```python
from build123d import *

# Parameters (mm, degrees)
SKETCH_1_R          = 6
EXTRUDE_1_DEPTH     = 19
CUT_EXTRUDE_1_DEPTH = 82.836727696


with BuildPart() as part:
    # Эскиз1 → Бобышка-Вытянуть1 (new, symmetric)
    with BuildSketch(Plane.XY):
        with BuildLine():
            Line((-31.8, 0), (-31.8, 16.2))
            ThreePointArc((-31.8, 16.2), (0, 48), (31.8, 16.2))
            Line((31.8, 16.2), (31.8, 0))
            Line((31.8, 0), (63.5, 0))
            Line((63.5, 0), (63.5, -14))
            Line((63.5, -14), (-63.5, -14))
            Line((-63.5, -14), (-63.5, 0))
            Line((-63.5, 0), (-31.8, 0))
        make_face()
        with Locations(Location((0, 16.2, 0), (0, 0, 180))):
            Circle(SKETCH_1_R, mode=Mode.SUBTRACT)
    extrude(amount=EXTRUDE_1_DEPTH, both=True)

    # Эскиз2 → Вырез-Вытянуть1 (cut, through all)
    with BuildSketch(Plane(origin=(0, 0, 0), x_dir=(1, 0, 0), z_dir=(0, 1, 0))):
        with BuildLine():
            Line((-51.5, 5), (-41.5, 5))
            ThreePointArc((-41.5, 5), (-36.5, 0), (-41.5, -5))
            Line((-41.5, -5), (-51.5, -5))
            ThreePointArc((-51.5, -5), (-56.5, 0), (-51.5, 5))
        make_face()
        with BuildLine():
            Line((51.5, 5), (41.5, 5))
            ThreePointArc((41.5, 5), (36.5, 0), (41.5, -5))
            Line((41.5, -5), (51.5, -5))
            ThreePointArc((51.5, -5), (56.5, 0), (51.5, 5))
        make_face()
    extrude(amount=-CUT_EXTRUDE_1_DEPTH, mode=Mode.SUBTRACT)


solid = part.part
```
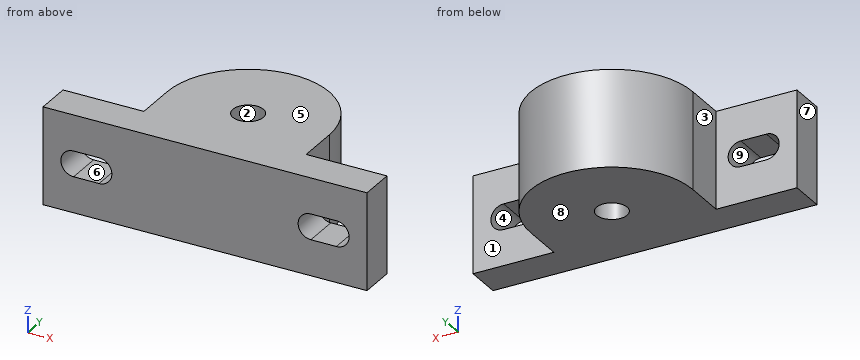
Check sheet for the modelled part. Datum: model origin and axes. Units: mm. Face numbers are marked on the shaded views. A direction names the side the tool comes from. Round coordinates to 2 decimals unless told otherwise and drop trailing zeros. Loops run counter-clockwise (first coordinate to the right, second up) from the corner with the lowest first, then second, coordinate; pieces in that order, holes last. Notation, with made-up numbers: (14.25, 84.5) - (25.25, 84.5) arc R30 cw to (25.25, 121.5) - close; hole circle Ø4 at (86.5, 74.25). An arc over 180 degrees is marked (long way). Answer as a JSON object with one key per item and string values. Group by question number.
Q1. Sectioned sample at A-A, the plane z = 0. Enter the section's corners in (x, y), plus the area to 3 significant figures.
Q2. Scan lines: line 1 along X through (y, z) = (16, 2); line 2 along Y through (x, z) = (0, -2); line 3 along X through (y, z) = (-3, -1.5). Record each from-to range of solid material in increasing order. Write a range as [from, to].
Q3. Sectioned sample at C-C, the plane z = 14. Enter the section's corners in (x, y), plus the area to 3 significant figures.
Q4. Set-up check for the marked faces 1, 2, 3, 4 and 5: record each of +Z, -Z, +X, -X, +Y, -Y from which the full face is reachable in a straight line by a thin tool's end or side.
Q5. Sectioned sample at D-D, the plane y = 13. Enter the section's corners in (x, z).
Q6. Sectioned sample at B-B, the plane x = 0. Enter the section's corners in (y, z), plus the area to 3 significant figures.
Q7. Mould release check, pull along Z, two halves, no side actions. Record for the marked faces 6, 7, 8 and 9: released by +Z, released by -Z, zero draft, split by the parting line, or undercut.
Q8. Gauge pin test, flat ends, axial feed: P1, Ø2, axis at y = 34.5, z = 6, coming from the +X side; P2, Ø12, axis at y = 30, z = -10.5, coming from the +X side; P3, Ø1, axis at x = -34, z = 14.5, coming from the +Y side. Record the tip position at first contact, or that the pin passes through.
Solution:
{
 "1": {"outline": "(-63.5, -14) - (-56.5, -14) - (-56.5, 0) - (-63.5, 0) - close; (-36.5, -14) - (36.5, -14) - (36.5, 0) - (31.8, 0) - (31.8, 16.2) arc R31.8 ccw to (-31.8, 16.2) - (-31.8, 0) - (-36.5, 0) - close; (56.5, -14) - (63.5, -14) - (63.5, 0) - (56.5, 0) - close; hole circle Ø12 at (0, 16.2)", "area": "3,720 mm²"},
 "2": {"line 1": "x = [-31.8, -6], [6, 31.8]", "line 2": "y = [-14, 10.2], [22.2, 48]", "line 3": "x = [-63.5, -56.27], [-36.73, 36.73], [56.27, 63.5]"},
 "3": {"outline": "(-63.5, -14) - (63.5, -14) - (63.5, 0) - (31.8, 0) - (31.8, 16.2) arc R31.8 ccw to (-31.8, 16.2) - (-31.8, 0) - (-63.5, 0) - close; hole circle Ø12 at (0, 16.2)", "area": "4,280 mm²"},
 "4": {"face 1": "+Z, -Z, +X, +Y", "face 2": "+Z, -Z", "face 3": "+Z, -Z, -X, +Y", "face 4": "+Y, -Y", "face 5": "+Z, +X, -X, +Y, -Y"},
 "5": {"outline": "(-31.8, -19) - (-5.08, -19) - (-5.08, 19) - (-31.8, 19) - close; (5.08, -19) - (31.8, -19) - (31.8, 19) - (5.08, 19) - close"},
 "6": {"outline": "(-14, -19) - (10.2, -19) - (10.2, 19) - (-14, 19) - close; (22.2, -19) - (48, -19) - (48, 19) - (22.2, 19) - close", "area": "1,900 mm²"},
 "7": {"face 6": "undercut", "face 7": "zero draft", "face 8": "released by -Z", "face 9": "undercut"},
 "8": {"P1": "stops at x = 26.68", "P2": "stops at x = 30.83", "P3": "stops at y = 0"}
}
